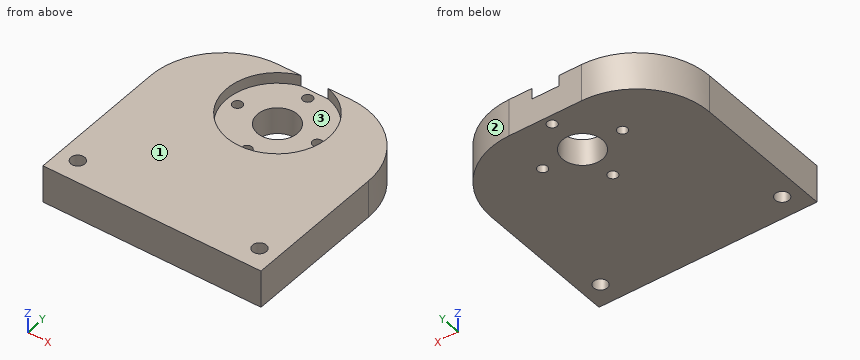
```python
from build123d import *

# Parameters (mm, degrees)
IZIM1_R                     = 1.9
IZIM1_R_2                   = 5.5
IZIM1_R_3                   = 1.35
Y_KSEKLIK_EKSTR_ZYON1_DEPTH = 10.3
IZIM2_R                     = 14
KES_EKSTR_ZYON1_DEPTH       = 3


with BuildPart() as part:
    # Çizim1 → Yükseklik-Ekstrüzyon1 (new body)
    with BuildSketch(Plane.XY):
        with BuildLine():
            Line((-15.927254298, -20.437118131), (44.072745702, -20.437118131))
            Line((44.072745702, -20.437118131), (44.072745702, 18.562881869))
            ThreePointArc((44.072745702, 18.562881869), (38.214881326, 32.705017493), (24.072745702, 38.562881869))
            Line((24.072745702, 38.562881869), (4.072745702, 38.562881869))
            ThreePointArc((4.072745702, 38.562881869), (-10.069389922, 32.705017493), (-15.927254298, 18.562881869))
            Line((-15.927254298, 18.562881869), (-15.927254298, -20.437118131))
        make_face()
        with Locations(Location((-10.927254298, -14.397118131, 0), (0, 0, 180))):
            Circle(IZIM1_R, mode=Mode.SUBTRACT)
        with Locations(Location((39.072745702, -14.397118131, 0), (0, 0, 180))):
            Circle(IZIM1_R, mode=Mode.SUBTRACT)
        with Locations(Location((14.072745702, 25.062881869, 0), (0, 0, 180))):
            Circle(IZIM1_R_2, mode=Mode.SUBTRACT)
        with Locations(Location((3.072745702, 25.062881869, 0), (0, 0, 180))):
            Circle(IZIM1_R_3, mode=Mode.SUBTRACT)
        with Locations(Location((14.072745702, 36.062881869, 0), (0, 0, 180))):
            Circle(IZIM1_R_3, mode=Mode.SUBTRACT)
        with Locations(Location((25.072745702, 25.062881869, 0), (0, 0, 180))):
            Circle(IZIM1_R_3, mode=Mode.SUBTRACT)
        with Locations(Location((14.072745702, 14.062881869, 0), (0, 0, 180))):
            Circle(IZIM1_R_3, mode=Mode.SUBTRACT)
    extrude(amount=Y_KSEKLIK_EKSTR_ZYON1_DEPTH)

    # Çizim2 → Kes-Ekstrüzyon1 (cut)
    with BuildSketch(Plane.XY.offset(10.3)):
        with Locations((14.072745702, 25.062881869)):
            Circle(IZIM2_R)
    extrude(amount=-KES_EKSTR_ZYON1_DEPTH, mode=Mode.SUBTRACT)


solid = part.part
```
For this review, take the finished solid that the model builds, in its own axes (mm). Face numbers are marked on the shaded views. Round coordinates to 2 decimals unless told otherwise and drop trailing zeros. Write each loop counter-clockwise with the first axis right and the second up, starting at its lowest first coordinate (ties: lowest second). Pieces come first, ordered by that corner, then holes. Notation, with made-up numbers: M 56.25,-27.75 L 89.25,-27.75 A18 cw 89.25,-15.75 Z; hole C 6,89 d3. An arc over 180 degrees is marked long. One line per item, written item: value. Start each with the question number.
(1) We need section D-D (x = 3). Give the boundary of the cut face in (y, z), and give its area (3 significant figures).
(2) We need section C-C (y = 17). Give the boundary of the cut face in (x, z), and give its area (3 significant figures).
(3) The part is to be moulded in two halves that separate along X. For the marked faces 1, 2 and 3, say which applies: released by +X, released by -X, zero draft, split by the parting line, or undercut.
(4) We need section A-A (x = 12). Give the boundary of the cut face in (y, z), and give its area (3 significant figures).
(5) Wall thickness on line 1 (Y direction, x = 26, z = 5.75); line 2 (Y direction, x = 18, z = 6); line 3 (Z direction, x = 16, y = 12): over which ranges is each line inside the solid? List them lowest first.
(6) We need section B-B (z = 6.25). Give the boundary of the cut face in (x, y).
(7) Insertion check: pin 1 (2 mm diameter, centred on x = 14.07, y = 36.06, fed in from -Z); pin 2 (17 mm diameter, centred on x = 14.07, y = 25.06, fed in from +Z); pin 3 (3 mm diameter, centred on y = 27.5, z = 3, fed in from +X). Each pin has a flat end and moves straight along its axis. Give the tip position at first contact, or say it passes through.
Result:
1. outline: M -20.44,0 L 23.71,0 L 23.71,7.3 L 16.5,7.3 L 16.5,10.3 L -20.44,10.3 Z; M 26.41,0 L 38.53,0 L 38.53,10.3 L 33.63,10.3 L 33.63,7.3 L 26.41,7.3 Z
1. area: 536 mm²
2. outline: M -15.93,0 L 44.07,0 L 44.07,10.3 L 25.52,10.3 L 25.52,7.3 L 2.63,7.3 L 2.63,10.3 L -15.93,10.3 Z
2. area: 549 mm²
3. face 1: zero draft
3. face 2: released by +X
3. face 3: undercut
4. outline: M -20.44,0 L 19.97,0 L 19.97,7.3 L 11.22,7.3 L 11.22,10.3 L -20.44,10.3 Z; M 30.16,0 L 38.56,0 L 38.56,7.3 L 30.16,7.3 Z
4. area: 451 mm²
5. line 1: -20.44 to 24.08, 26.04 to 38.47
5. line 2: -20.44 to 21.21, 28.91 to 38.56
5. line 3: 0 to 7.3
6. outline: M -15.93,-20.44 L 44.07,-20.44 L 44.07,18.56 A20 ccw 24.07,38.56 L 4.07,38.56 A20 ccw -15.93,18.56 Z; hole C -10.93,-14.4 d3.8; hole C 3.07,25.06 d2.7; hole C 14.07,25.06 d11; hole C 14.07,14.06 d2.7; hole C 14.07,36.06 d2.7; hole C 25.07,25.06 d2.7; hole C 39.07,-14.4 d3.8
7. pin 1: through
7. pin 2: z = 7.3
7. pin 3: x = 42.64
